The listing builds one solid part. Answer for the finished solid, in the listing's coordinates (mm). Face numbers are marked on the shaded views. A direction names the side the tool comes from. Coordinates: 2 decimals unless noted, no trailing zeros. Order: outer loops, then holes, each group sorted by start corner. A loop starts at its lowest first (then second) coordinate and runs counter-clockwise, first axis right, second up.
Autodesk Fusion 360 part; units mm, degrees
sketch "Sketch1" plane through (0, 0, 0) normal (0, 0, 1) x (1, 0, 0)
  circle A0 centre (-43, 0) radius 19
  circle A1 centre (-43, 0) radius 9.5
  line L0 (-37, 44) -> (-37, 18.0278)
  line L1 (-37, -44) -> (-37, -18.0278)
  line L2 (-37, -44) -> (43, -44)
  line L3 (-37, 44) -> (43, 44)
  line L4 (-37, 44) -> (-24, 44)
  line L5 (-24, 0) -> (-21, 0)
  line L6 (-21, 19) -> (-24, 19)
  line L7 (-21, -19) -> (-24, -19)
  line L8 (-24, 19) -> (-24, 44)
  line L9 (-24, -19) -> (-24, -44)
  line L10 (-21, 0) -> (-17, 0)
  line L11 (-17, 0) -> (-17, 5)
  line L12 (-17, 0) -> (-17, -5)
  line L13 (-17, 5) -> (-21, 5)
  line L14 (-17, -5) -> (-21, -5)
  line L15 (-21, -5) -> (-21, -19)
  line L16 (-21, 5) -> (-21, 19)
  circle A2 centre (7, 25) radius 5
  circle A3 centre (7, -25) radius 5
  line L17 (43, 44) -> (62, 44)
  line L18 (62, 44) -> (62, -44)
  line L19 (43, -44) -> (62, -44)
  dimension "d8" = 13
  dimension "d21" = 19
  dimension "d22" = 88
extrude "Extrude1" add sketch "Sketch1" along normal blind 50 contours A0 | A0 L1 L2 L5 L7 L9 L10 L12 L14 L15 | A0 L0 L3 L4 L5 L6 L8 L10 L11 L13 L16
extrude "Extrude2" add sketch "Sketch1" along normal blind 10 contours L2 L3 L6 L7 L8 L9 L11 L12 L13 L14 L15 L16 L17 L18 L19
chamfer "Chamfer1" distance 36.5 angle 45 2 edges at (62, -44, 5) (62, 44, 5)
fillet "Fillet1" radius 19 2 edges at (62, -7.5, 5) (62, 7.5, 5)
fillet "Fillet2" radius 13 1 edges at (25.5, -44, 5)
fillet "Fillet3" radius 13 1 edges at (25.5, 44, 5)
fillet "Fillet4" radius 3 1 edges at (-24, -19, 30)
fillet "Fillet5" radius 3 1 edges at (-24, 19, 30)
fillet "Fillet6" radius 6 1 edges at (-37, 18.0278, 25)
fillet "Fillet7" radius 6 1 edges at (-37, -18.0278, 25)
sketch "Sketch2" plane through (0, 0, 0) normal (0, 1, 0) x (1, 0, 0)
  line L0 (-17.1305, -49.9822) -> (-17.1305, -10.123)
  line L1 (-17.1305, -10.123) -> (49.8695, -10.123)
  line L2 (-17.1305, -49.9822) -> (49.8695, -10.123)
  dimension "d42" = 67
extrude "Extrude3" add sketch "Sketch2" along normal mid plane 10
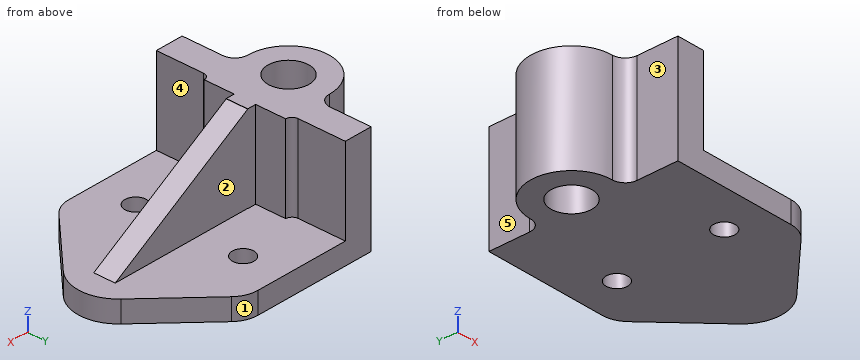
1) Section D-D (y = -28.5) is taken. Give the vertices of the cut face in (x, z).
2) Consider L1, parallel to Y at x = 7, z = 5.5; L2, parallel to Y at x = -43, z = 30; L3, parallel to Y at x = -6.5, z = 22. Determine where each line is inside the solid, lowest interval first.
3) Each of these flat-tipped pins is pushed along its axis until it touches: P1, Ø2, axis at y = -2, z = 22, coming from the -X side; P2, Ø7, axis at y = 14.5, z = 36, coming from the +X side; P3, Ø5, axis at x = 17.5, z = 30.5, coming from the -Y side. Where does it stop, or does it pass through?
4) Section A-A (x = 7) is taken. Give the vertices of the cut face in (y, z).
5) Section C-C (x = -35.5) is taken. Give the vertices of the cut face in (y, z).
6) A tool of negligible diameter and unlimited length cuts with its end or side. For the marked faces 1, 2, 3, 4 and 5, from which of +Z, -Z, +X, -X, +Y, -Y can it reach the whole face along a straight path? Write none if from no direction.
Filled sheet:
1. outline: (-37, 0) - (3.43, 0) - (3.43, 10) - (-24, 10) - (-24, 50) - (-37, 50) - close; (10.57, 0) - (41, 0) - (41, 10) - (10.57, 10) - close
2. L1: y = -44 to -30, -20 to 20, 30 to 44
2. L2: y = -19 to -9.5, 9.5 to 19
2. L3: y = -5 to 5
3. P1: stops at x = -61.97
3. P2: stops at x = -21
3. P3: stops at y = -5
4. outline: (-44, 0) - (-30, 0) - (-30, 10) - (-44, 10) - close; (-20, 0) - (20, 0) - (20, 10) - (-20, 10) - close; (-5, 10.12) - (5, 10.12) - (5, 35.63) - (-5, 35.63) - close; (30, 0) - (44, 0) - (44, 10) - (30, 10) - close
5. outline: (-44, 0) - (-5.83, 0) - (-5.83, 50) - (-44, 50) - close; (5.83, 0) - (44, 0) - (44, 50) - (5.83, 50) - close
6. face 1: +Z, -Z, +X, +Y
6. face 2: +Z, +X, +Y
6. face 3: +Z, -Z, -X, -Y
6. face 4: +Z, +X, -Y
6. face 5: +Z, -Z, -X, +Y
